Part model, mm, in its own coordinate system. Round coordinates to 2 decimals unless told otherwise and drop trailing zeros. Write each loop counter-clockwise with the first axis right and the second up, starting at its lowest first coordinate (ties: lowest second). Pieces come first, ordered by that corner, then holes. Notation, with made-up numbers: M 60.25,29.25 L 68.25,29.25 A7 cw 68.25,36.25 Z; hole C 47,28 d7. An arc over 180 degrees is marked long. Use a Markdown table: item, result. Add a question column.
1) Two-plate mould, pull along Z, no slides. Class faces 1 (the face through (263, 0, -304)), 2 (the face through (470.476, 1.479, -25.664)): released by +Z, released by -Z, zero draft, split by the parting line, or undercut.
2) Drop flat-ended pins along their axis: P1, Ø0.9, axis at y = 1, z = 5, coming from the -X side; P2, Ø1.5, axis at x = 4.5, y = 2, coming from the -Z side; P3, Ø1.5, axis at x = 4, y = 1.5, coming from the +Z side. Give the stop position or say it passes through.
3) Slice it at A-A on x = 490. Write the cut outline in (y, z), plus the area to 3 significant figures.
4) Slice it at B-B on z = -30. Write the cut outline in (x, y), plus the area to 3 significant figures.
5) Wall check: probe 1 along X at (y, z) = (1.25, -530). Give the ranges that are in metal, low to high.
```python
from build123d import *

# Parameters (mm, degrees)
SKETCH1_W           = 534
SKETCH1_H           = 600
BOSS_EXTRUDE1_DEPTH = 3
SKETCH3_W           = 520
SKETCH3_H           = 614
BOSS_EXTRUDE2_DEPTH = 3
SKETCH4_R           = 20
CUT_EXTRUDE5_DEPTH  = 10
SKETCH5_R           = 20
CUT_EXTRUDE7_DEPTH  = 10


with BuildPart() as part:
    # Sketch1 → Boss-Extrude1 (new body)
    with BuildSketch(Plane(origin=(0, 0, 0), x_dir=(1, 0, 0), z_dir=(0, 1, 0))):
        with Locations((267.046520854, 300.291126183)):
            Rectangle(SKETCH1_W, SKETCH1_H)
    extrude(amount=BOSS_EXTRUDE1_DEPTH)

    # Sketch3 → Boss-Extrude2 (add)
    with BuildSketch(Plane(origin=(0, 0, 0), x_dir=(1, 0, 0), z_dir=(0, 1, 0))):
        with Locations((267, 300)):
            Rectangle(SKETCH3_W, SKETCH3_H)
    extrude(amount=BOSS_EXTRUDE2_DEPTH)

    # Sketch4 → Cut-Extrude5 (cut)
    with BuildSketch(Plane(origin=(0, 3, 0), x_dir=(1, 0, 0), z_dir=(0, 1, 0))):
        with Locations(Location((490, 530, 0), (0, 0, 270))):
            Circle(SKETCH4_R)
    extrude(amount=-CUT_EXTRUDE5_DEPTH, mode=Mode.SUBTRACT)

    # Sketch5 → Cut-Extrude7 (cut)
    with BuildSketch(Plane(origin=(0, 0, 0), x_dir=(-1, 0, 0), z_dir=(0, -1, 0))):
        with Locations(Location((-490, 30, 0), (0, 0, 90))):
            Circle(SKETCH5_R)
    extrude(amount=-CUT_EXTRUDE7_DEPTH, mode=Mode.SUBTRACT)


solid = part.part
```
Entries:
| question | item | result |
|---|---|---|
| 1 | face 1 | zero draft |
| 1 | face 2 | undercut |
| 2 | P1 | stops at x = 7 |
| 2 | P2 | stops at z = -600.29 |
| 2 | P3 | stops at z = -0.29 |
| 3 | outline | M 0,-607 L 3,-607 L 3,-550 L 0,-550 Z; M 0,-510 L 3,-510 L 3,-50 L 0,-50 Z; M 0,-10 L 3,-10 L 3,7 L 0,7 Z |
| 3 | area | 1,600 mm^2 |
| 4 | outline | M 0.05,0 L 470,0 L 470,3 L 0.05,3 Z; M 510,0 L 534.05,0 L 534.05,3 L 510,3 Z |
| 4 | area | 1,480 mm^2 |
| 5 | probe 1 | x = 0.05 to 470, 510 to 534.05 |
